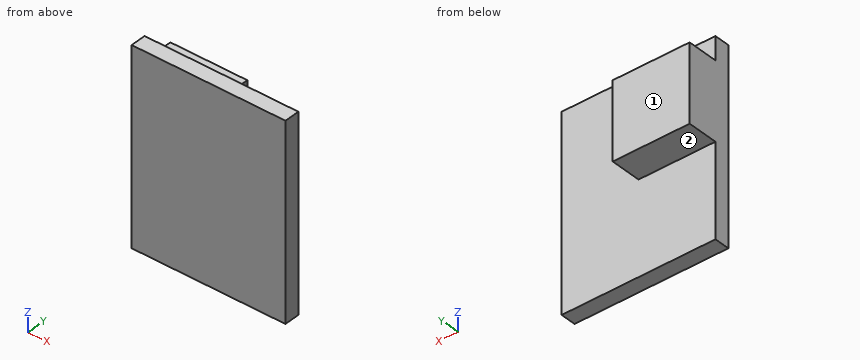
Autodesk Inventor part; units mm, degrees
ref_plane "YZ Plane" through (0, 0, 0) normal (1, 0, 0) x (0, 1, 0)
ref_plane "XZ Plane" through (0, 0, 0) normal (0, 1, 0) x (-1, 0, 0)
ref_plane "XY Plane" through (0, 0, 0) normal (0, 0, 1) x (1, 0, 0)
sketch "Sketch1" plane through (0, 0, 0) normal (0, 1, 0) x (-1, 0, 0)
  line L0 (-10, 12.5) -> (10, 12.5)
  line L1 (10, 12.5) -> (10, -12.5)
  line L2 (10, -12.5) -> (-10, -12.5)
  line L3 (-10, -12.5) -> (-10, 12.5)
  line L4 (-10, 12.5) -> (10, -12.5) construction
  line L5 (10, 12.5) -> (-10, -12.5) construction
  point P0 (0, 0)
  dimension "d0" = 20
  dimension "d1" = 25
extrude "Extrusion1" add sketch "Sketch1" along normal blind 2
sketch "Sketch2" plane through (0, 2, 0) normal (0, 1, 0) x (1, 0, 0)
  line L0 (-10, -9.5) -> (0, -9.5)
  line L1 (0, -9.5) -> (0, 0.5)
  line L2 (0, 0.5) -> (-10, 0.5)
  line L3 (-10, 0.5) -> (-10, -9.5)
  point P0 (0, 0)
  dimension "d4" = 10
  dimension "d5" = 10
extrude "Extrusion2" add sketch "Sketch2" along normal blind 4
properties part number "POWER_DELIVERY"
Geometry: final body of the model. Coordinates: model frame, mm. Face numbers are marked on the shaded views. A direction names the side the tool comes from. Coordinates: 2 decimals unless noted, no trailing zeros. Loops run counter-clockwise (first coordinate to the right, second up) from the corner with the lowest first, then second, coordinate; pieces in that order, holes last. Notation, with made-up numbers: (2, 4) - (38, 4) arc R23 cw to (38, 37) - close; hole circle Ø2 at (-8, 79.25). An arc over 180 degrees is marked (long way). One line per question, with ' | ' between items. Start each with the question number.
(1) Reachability of the marked faces 1 and 2 from +Z, -Z, +X, -X, +Y, -Y: full face, straight path, thin tool, end or side. Return the list, or none.
(2) Cut plane D-D on z = -5. Output: boundary loops of the cut face in (x, y).
(3) Ray query, L1, parallel to X at y = 3, z = 1.75; L2, parallel to Y at x = -2.25, z = -1; L3, parallel to Z at x = -4.25, y = 2.05. Return the intervals inside material, ascending. Write a range as from..to.
(4) First-contact query: pin 1 (1.2 mm diameter, centred on y = 3.5, z = 7, fed in from +X); pin 2 (2 mm diameter, centred on x = -7.5, y = 2.5, fed in from -Z); pin 3 (1 mm diameter, centred on x = -4, z = -4.5, fed in from +Y); pin 4 (1.2 mm diameter, centred on x = -6.5, y = 4.5, fed in from -Z). Flat tips, straight axial feed; report the tip coordinate or a pass-through.
(5) Cut plane A-A on x = -5.5. Output: boundary loops of the cut face in (y, z).
(6) Cut plane C-C on z = 4.5. Output: boundary loops of the cut face in (x, y), and give its area (3 significant figures).
(7) Cut plane B-B on y = 5.1. Output: boundary loops of the cut face in (x, z).
Here are the results:
1) face 1: +Z, -Z, +X, -X, +Y | face 2: -Z, +X, -X, +Y
2) outline: (-10, 0) - (10, 0) - (10, 2) - (-10, 2) - close
3) L1: -10..0 | L2: 0..2 | L3: -0.5..9.5
4) pin 1: x = 0 | pin 2: z = -12.5 | pin 3: y = 2 | pin 4: z = -0.5
5) outline: (0, -12.5) - (2, -12.5) - (2, -0.5) - (6, -0.5) - (6, 9.5) - (2, 9.5) - (2, 12.5) - (0, 12.5) - close
6) outline: (-10, 0) - (10, 0) - (10, 2) - (0, 2) - (0, 6) - (-10, 6) - close | area: 80.0 mm²
7) outline: (-10, -0.5) - (0, -0.5) - (0, 9.5) - (-10, 9.5) - close
